```python
from build123d import *

# Parameters (mm, degrees)
BOSS_EXTRUDE1_DEPTH             = 3.175
M3X0_5_TAPPED_HOLE1_D           = 2.5
M3X0_5_TAPPED_HOLE1_CSINK_D     = 3.05
M3X0_5_TAPPED_HOLE1_CSINK_ANGLE = 90


with BuildPart() as part:
    # Sketch1 → Boss-Extrude1 (new body)
    with BuildSketch(Plane(origin=(0, 0, 0), x_dir=(1, 0, 0), z_dir=(0, 1, 0))):
        Polygon((0, 86.763269807), (-10, 85), (-10, 115), (0, 113.236730193), (0, 200), (-250, 200), (-250, -200), (0, -200), (0, -113.236730193), (10, -115), (10, -85), (0, -86.763269807), align=None)
    extrude(amount=BOSS_EXTRUDE1_DEPTH)

    # M3x0.5 Tapped Hole1 (through all)
    with Locations(Plane(origin=(0, 3.175, 0), x_dir=(1, 0, 0), z_dir=(0, 1, 0))):
        with Locations((-193.539921074, 142.5), (-193.539921074, -142.5), (-54.516495305, 142.5), (-54.516495305, -142.5), (-242.5, -170), (-242.5, 170), (-7.5, -170), (-7.5, 170)):
            CounterSinkHole(M3X0_5_TAPPED_HOLE1_D / 2, M3X0_5_TAPPED_HOLE1_CSINK_D / 2, counter_sink_angle=M3X0_5_TAPPED_HOLE1_CSINK_ANGLE)


solid = part.part
```
Model file for the job. Use its own axes, mm. Coordinates: 2 decimals unless noted, no trailing zeros. Order: outer loops, then holes, each group sorted by start corner. A loop starts at its lowest first (then second) coordinate and runs counter-clockwise, first axis right, second up. Notation, with made-up numbers: (-0.5, 45) - (16.5, 45) arc R28 cw to (16.5, 73) - close; hole circle Ø4 at (81, 57.5). An arc over 180 degrees is marked (long way). Return JSON: item names as keys, results as strings. Group by question number.
1) Probe line 1 (X direction, y = 1.4, z = -170); line 2 (Z direction, x = -242.5, y = 2.05); line 3 (X direction, y = 0.8, z = -142.5). List the from-to ranges inside material, lowest first. Write a range as from..to.
2) Saw through at A-A, the plane y = 0.65. Count the separate pieces of the cut face and the enclosed holes in it, plus the area to 4 significant figures.
3) Flat gauge pins, fed straight in: P1, Ø1, axis at y = 1, z = 168.5, coming from the +X side; P2, Ø3, axis at x = -242.5, z = -170, coming from the -Y side; P3, Ø1, axis at y = 1.5, z = -98, coming from the +X side. Where does each tip first touch, or does it go through?
4) Saw through at B-B, the plane z = 3. Write the cut outline in (x, y) (3 decimals).
Values found:
{
 "1": {"line 1": "x = -250..-243.75, -241.25..-8.75, -6.25..0", "line 2": "z = -200..-171.25, -168.75..168.75, 171.25..200", "line 3": "x = -250..-194.79, -192.29..-55.77, -53.27..0"},
 "2": {"separate pieces": "1", "enclosed holes": "8", "area": "100,000 mm²"},
 "3": {"P1": "stops at x = 0", "P2": "stops at y = 0", "P3": "stops at x = -10"},
 "4": {"outline": "(-250, 0) - (0, 0) - (0, 3.175) - (-250, 3.175) - close"}
}
